```python
from build123d import *

# Parameters (mm, degrees)
BOSS_EXTRUDE1_DEPTH = 5
SKETCH2_W           = 3
SKETCH2_H           = 30
BOSS_EXTRUDE2_DEPTH = 30
FILLET1_R           = 10
BOSS_EXTRUDE3_DEPTH = 3.5
BOSS_EXTRUDE4_DEPTH = 3.5
FILLET2_R           = 1


with BuildPart() as part:
    # Sketch1 → Boss-Extrude1 (new body)
    with BuildSketch(Plane(origin=(0, 0, 0), x_dir=(1, 0, 0), z_dir=(0, 1, 0))):
        with BuildLine():
            Line((5, 0), (65, 0))
            ThreePointArc((65, 0), (68.535533906, 1.464466094), (70, 5))
            Line((70, 5), (70, 35))
            ThreePointArc((70, 35), (68.535533906, 38.535533906), (65, 40))
            Line((65, 40), (5, 40))
            ThreePointArc((5, 40), (1.464466094, 38.535533906), (0, 35))
            Line((0, 35), (0, 5))
            ThreePointArc((0, 5), (1.464466094, 1.464466094), (5, 0))
        make_face()
    extrude(amount=BOSS_EXTRUDE1_DEPTH)

    # Sketch2 → Boss-Extrude2 (add)
    with BuildSketch(Plane.XZ):
        with Locations((1.5, -20)):
            Rectangle(SKETCH2_W, SKETCH2_H)
        with Locations((68.5, -20)):
            Rectangle(SKETCH2_W, SKETCH2_H)
    extrude(amount=BOSS_EXTRUDE2_DEPTH)

    # Fillet1
    # the kernel refuses this fillet: 10 mm, written as the material it takes off along each edge
    with BuildSketch(Plane(origin=(0, -30, -52.853571071), x_dir=(0, 1, 0), z_dir=(0, 0, 1))) as fillet1_piece_1:
        with BuildLine():
            CenterArc((7.141428429, -10), FILLET1_R, 90, 45.572995999)
            Line((0, -3), (-0.142828569, -2.86))
            ThreePointArc((-0.142828569, -2.86), (-0.2, -1.5), (-0.2, 0))
            Line((-0.2, 0), (0, 0.2))
            Line((0, 0.2), (7.141428429, 0.2))
            Line((7.141428429, 0.2), (7.141428429, 0))
        make_face()
    extrude(amount=65.707142143, mode=Mode.SUBTRACT)
    with BuildSketch(Plane(origin=(70, -30, -52.853571071), x_dir=(0, 1, 0), z_dir=(0, 0, 1))) as fillet1_piece_2:
        with BuildLine():
            CenterArc((7.141428429, 10), FILLET1_R, 224.427004001, 45.572995999)
            Line((0, 3), (-0.142828569, 2.86))
            ThreePointArc((-0.142828569, 2.86), (-0.2, 1.5), (-0.2, 0))
            Line((-0.2, 0), (0, -0.2))
            Line((0, -0.2), (7.141428429, -0.2))
            Line((7.141428429, -0.2), (7.141428429, 0))
        make_face()
    extrude(amount=65.707142143, mode=Mode.SUBTRACT)

    # Sketch3 → Boss-Extrude3 (add)
    with BuildSketch(Plane.ZY.offset(-15)):
        Polygon((-25, 7.5), (-31.5, 7.5), (-31.5, 32.5), (-28, 32.5), (-31.5, 42.5), (-31.5, 54.5), (-40, 54.5), (-40, 5), (0, 5), (0, 17.5), (-4, 17.5), (-4, 7.5), (-15, 7.5), (-15, 11), (-25, 11), align=None)
    extrude(amount=BOSS_EXTRUDE3_DEPTH)

    # Sketch4 → Boss-Extrude4 (add)
    with BuildSketch(Plane.ZY.offset(-55)):
        with BuildLine():
            Line((-31.5, 7.5), (-31.5, 32.5))
            Line((-31.5, 32.5), (-28, 32.5))
            Line((-28, 32.5), (-31.5, 42.5))
            Line((-31.5, 42.5), (-31.5, 54.5))
            Line((-31.5, 54.5), (-40, 54.5))
            Line((-40, 54.5), (-40, 5))
            Line((-40, 5), (0, 5))
            Line((0, 5), (0, 0))
            ThreePointArc((0, 0), (5.624620047, 2.01707195), (8, 7.5))
            Line((8, 7.5), (8, 17.5))
            Line((8, 17.5), (3, 17.5))
            Line((3, 17.5), (3, 7.5))
            Line((3, 7.5), (-15, 7.5))
            Line((-15, 7.5), (-15, 11))
            Line((-15, 11), (-25, 11))
            Line((-25, 11), (-25, 7.5))
            Line((-25, 7.5), (-31.5, 7.5))
        make_face()
    extrude(amount=-BOSS_EXTRUDE4_DEPTH)

    # Fillet2
    fillet2_edges = [part.edges().sort_by_distance(p)[0] for p in [
        (56.75, 17.5, 3),
        (56.75, 17.5, 8),
        (56.75, 54.5, -40),
        (56.75, 54.5, -31.5),
        (56.75, 32.5, -28),
        (13.25, 54.5, -31.5),
        (13.25, 54.5, -40),
        (13.25, 17.5, 0),
        (13.25, 17.5, -4),
        (13.25, 11, -15),
        (13.25, 11, -25),
        (13.25, 32.5, -28),
        (56.75, 11, -25),
        (56.75, 11, -15),
    ]]
    fillet(fillet2_edges, radius=FILLET2_R)


solid = part.part
```
CAD build for the part. Positions are in the model's coordinates, mm. A direction names the side the tool comes from. Give positions to 0.01 mm unless a question says otherwise; leave off trailing zeros. Order: outer loops, then holes, each group sorted by start corner. A loop starts at its lowest first (then second) coordinate and runs counter-clockwise, first axis right, second up.
(1) Drill centre lines: L1, parallel to X at y = -19, z = -11; L2, parallel to X at y = 6, z = -10.5; L3, parallel to Y at x = 20, z = -3. Where is each one in solid material? Low to high.
(2) Saw through at A-A, the plane y = 48. Give the cut face in (x, z).
(3) Saw through at C-C, the plane z = -6. Give the cut face in (x, y).
(4) Saw through at B-B, the plane z = -30.5. Give the cut face in (x, y).
(5) Mould opens along Z. For faces 5 (the flat face through (13, 11, -20)), 6 (the flat face through (15, 24, -32)), 7 (the flat face through (57, 48, -31.5)) say: released by +Z, released by -Z, zero draft, split by the parting line, or undercut.
(6) Flat gauge pins, fed straight in: pin 1 (1.8 mm diameter, centred on x = 12.5, y = 19, fed in from +Z); pin 2 (2 mm diameter, centred on y = 18.5, z = -35, fed in from -X); pin 3 (2 mm diameter, centred on x = 18, z = -14.5, fed in from +Y); pin 4 (14.5 mm diameter, centred on y = 37.5, z = -19.5, fed in from -X). Where does each tip first touch, or does it go through?
(7) Tool access for faces 1 (the flat face through (68, -15, -35)), 2 (the flat face through (6, 5, -20)), 3 (the flat face through (13, 48, -31.5)), 4 (the flat face through (57, 9, -25)): list every direction of +Z, -Z, +X, -X, +Y, -Y with a clear straight run to the whole face (end or side of a thin tool).
(8) Saw through at D-D, the plane y = -20. Give the cut face in (x, z), then the cut area to 3 significant figures.
Results found:
1. L1: x = 0 to 3, 67 to 70
1. L2: x = 11.5 to 15, 55 to 58.5
1. L3: y = 0 to 5
2. outline: (11.5, -40) - (15, -40) - (15, -31.5) - (11.5, -31.5) - close; (55, -40) - (58.5, -40) - (58.5, -31.5) - (55, -31.5) - close
3. outline: (0, -22.86) arc R10 ccw to (3, -30) - (3, 0) - (67, 0) - (67, -30) arc R10 ccw to (70, -22.86) - (70, 5) - (58.5, 5) - (58.5, 7.5) - (55, 7.5) - (55, 5) - (15, 5) - (15, 7.5) - (11.5, 7.5) - (11.5, 5) - (0, 5) - close
4. outline: (0, -22.86) arc R10 ccw to (3, -30) - (3, 0) - (67, 0) - (67, -30) arc R10 ccw to (70, -22.86) - (70, 5) - (58.5, 5) - (58.5, 7.5) - (55, 7.5) - (55, 5) - (15, 5) - (15, 7.5) - (11.5, 7.5) - (11.5, 5) - (0, 5) - close; (11.5, 32.5) - (15, 32.5) - (15, 39.64) - (11.5, 39.64) - close; (55, 32.5) - (58.5, 32.5) - (58.5, 39.64) - (55, 39.64) - close
5. face 5: undercut
5. face 6: zero draft
5. face 7: released by +Z
6. pin 1: stops at z = -31.5
6. pin 2: stops at x = 11.5
6. pin 3: stops at y = 5
6. pin 4: passes through
7. face 1: -Z, +X, -X, -Y
7. face 2: +Z, -Z, -X, +Y
7. face 3: +Z, +X, -X, +Y
7. face 4: +X, -X, +Y
8. outline: (0, -35) - (3, -35) - (3, -5) - (0, -5) - close; (67, -35) - (70, -35) - (70, -5) - (67, -5) - close
8. area: 180 mm2
